Part model, mm, in its own coordinate system. Give positions to 0.01 mm unless a question says otherwise; leave off trailing zeros. Order: outer loops, then holes, each group sorted by start corner. A loop starts at its lowest first (then second) coordinate and runs counter-clockwise, first axis right, second up.
1. Mould opens along X. For faces 1 (the flat face through (-3, -7, 0)), 2 (the cylindrical face through (-4.931, 8.136, 0.74)), 3 (the cylindrical face through (36, -9.76, 0.74)) say: +X half, -X half, draft (parallel to the pull), parting line (faces both ways), or undercut.
2. Slice it at C-C on x = -1.5. List the corners of the cut face in (y, z).
3. Slice it at D-D on z = 0.4. Give the number of separate pieces and of enclosed holes in the cut face, and give its area (3 significant figures).
4. Probe line 1 (Y direction, x = 5, z = 0.65); line 2 (Y direction, x = 7.5, z = 0.5); line 3 (X direction, y = -2, z = 1.05). List the from-to ranges inside material, lowest first.
5. Slice it at A-A on x = 5. List the corners of the cut face in (y, z).
6. Slice it at B-B on y = 0. List the corners of the cut face in (x, z), and give its area (3 significant figures).
Autodesk Inventor part; units mm, degrees
ref_plane "YZ Plane" through (0, 0, 0) normal (1, 0, 0) x (0, 1, 0)
ref_plane "XZ Plane" through (0, 0, 0) normal (0, 1, 0) x (-1, 0, 0)
ref_plane "XY Plane" through (0, 0, 0) normal (0, 0, 1) x (1, 0, 0)
sketch "スケッチ1" plane through (0, 0, 0) normal (0, 0, 1) x (1, 0, 0)
  line L0 (25, -23) -> (-25, -23) construction
  line L1 (25, 23) -> (25, -23) construction
  line L2 (-25, 23) -> (25, 23) construction
  arc A0 (8.5, 1.9365) -> (7.0484, 3.4357) centre (7, 1.9365) ccw construction
  line L3 (8.5, 1.9365) -> (8.5, -1.9365) construction
  arc A1 (7.0484, -3.4357) -> (8.5, -1.9365) centre (7, -1.9365) ccw construction
  arc A2 (2.9516, -3.4357) -> (7.0484, -3.4357) centre (5, 0) ccw construction
  arc A3 (1.5, -1.9365) -> (2.9516, -3.4357) centre (3, -1.9365) ccw construction
  line L4 (1.5, -1.9365) -> (1.5, 1.9365) construction
  arc A4 (2.9516, 3.4357) -> (1.5, 1.9365) centre (3, 1.9365) ccw construction
  arc A5 (7.0484, 3.4357) -> (2.9516, 3.4357) centre (5, 0) ccw construction
  circle A6 centre (5, 0) radius 27.5 construction
  circle A7 centre (5, 0) radius 15.5 construction
  circle A8 centre (5, 0) radius 13.75 construction
  line L5 (25, 14) -> (25, 23) construction
  line L6 (-275, 23) -> (25, 23) construction
  line L7 (-275, 23) -> (-275, 14)
  line L8 (-275, 14) -> (25, 14) construction
  line L9 (25, -23) -> (25, -14) construction
  line L10 (-275, -14) -> (25, -14) construction
  line L11 (-275, -14) -> (-275, -23)
  line L12 (-275, -23) -> (25, -23) construction
  circle A9 centre (18.75, 0) radius 1.6
  circle A10 centre (14.7227, 9.7227) radius 1.6
  circle A11 centre (5, 13.75) radius 1.6
  circle A12 centre (-4.7227, 9.7227) radius 1.6
  circle A13 centre (-8.75, 0) radius 1.6
  circle A14 centre (-4.7227, -9.7227) radius 1.6
  circle A15 centre (5, -13.75) radius 1.6
  circle A16 centre (14.7227, -9.7227) radius 1.6
  circle A17 centre (5, 0) radius 10
  circle A18 centre (5, 0) radius 32.5
  point P0 (0, 0)
  dimension "d3" = 27.5
  dimension "d1" = 55
  dimension "d2" = 31
  dimension "d4" = 3.2
  dimension "d7" = 360
  dimension "d9" = 20
  dimension "d12" = 65
extrude "押し出し1" add sketch "スケッチ1" along normal blind 1.5
properties part number "先端アームパーツA" material "アルミニウム 6061"
Data:
1. face 1: draft
1. face 2: undercut
1. face 3: parting line
2. outline: (-31.84, 0) - (-7.6, 0) - (-7.6, 1.5) - (-31.84, 1.5) - close; (7.6, 0) - (31.84, 0) - (31.84, 1.5) - (7.6, 1.5) - close
3. separate pieces: 1
3. enclosed holes: 9
3. area: 2,940 mm2
4. line 1: y = -32.5 to -15.35, -12.15 to -10, 10 to 12.15, 15.35 to 32.5
4. line 2: y = -32.4 to -9.68, 9.68 to 32.4
4. line 3: x = -27.44 to -4.8, 14.8 to 37.44
5. outline: (-32.5, 0) - (-15.35, 0) - (-15.35, 1.5) - (-32.5, 1.5) - close; (-12.15, 0) - (-10, 0) - (-10, 1.5) - (-12.15, 1.5) - close; (10, 0) - (12.15, 0) - (12.15, 1.5) - (10, 1.5) - close; (15.35, 0) - (32.5, 0) - (32.5, 1.5) - (15.35, 1.5) - close
6. outline: (-27.5, 0) - (-10.35, 0) - (-10.35, 1.5) - (-27.5, 1.5) - close; (-7.15, 0) - (-5, 0) - (-5, 1.5) - (-7.15, 1.5) - close; (15, 0) - (17.15, 0) - (17.15, 1.5) - (15, 1.5) - close; (20.35, 0) - (37.5, 0) - (37.5, 1.5) - (20.35, 1.5) - close
6. area: 57.9 mm2
